Check sheet for the modelled part. Datum: model origin and axes. Units: mm. Face numbers are marked on the shaded views. A direction names the side the tool comes from. Round coordinates to 2 decimals unless told otherwise and drop trailing zeros. Write each loop counter-clockwise with the first axis right and the second up, starting at its lowest first coordinate (ties: lowest second). Pieces come first, ordered by that corner, then holes. Notation, with made-up numbers: (70.25, 2) -> (102.25, 2) arc R16 cw to (102.25, 20) -> close; hole circle Ø11 at (-34.75, 31). An arc over 180 degrees is marked (long way). Put each result on its own line as item: value. Start each with the question number.
from build123d import *

# Parameters (mm, degrees)
BOSS_EXTRUDE1_DEPTH                             = 6.35
SKETCH2_R                                       = 16.256
CUT_EXTRUDE1_DEPTH                              = 7.62
SKETCH3_R                                       = 10
CUT_EXTRUDE2_DEPTH                              = 31.770069873
CSK_FOR_M3_FLAT_HEAD_MACHINE_SCREW1_D           = 3.4
CSK_FOR_M3_FLAT_HEAD_MACHINE_SCREW1_CSINK_D     = 6.3
CSK_FOR_M3_FLAT_HEAD_MACHINE_SCREW1_CSINK_ANGLE = 90
CIRPATTERN1_COUNT                               = 4
F_8_32_TAPPED_HOLE1_D                           = 3.4544
F_8_32_TAPPED_HOLE1_DEPTH                       = 12.7
F_8_32_TAPPED_HOLE1_TIP                         = 1.037806461


with BuildPart() as part:
    # Sketch1 → Boss-Extrude1 (new, symmetric)
    with BuildSketch(Plane.XY):
        with BuildLine():
            Line((-21.08, 0), (-21.08, -17.78))
            Line((-21.08, -17.78), (21.08, -17.78))
            Line((21.08, -17.78), (21.08, 0))
            ThreePointArc((21.08, 0), (0, 21.08), (-21.08, 0))
        make_face()
    extrude(amount=BOSS_EXTRUDE1_DEPTH, both=True)

    # Sketch2 → Cut-Extrude1 (cut)
    with BuildSketch(Plane.XY.offset(6.35)):
        Circle(SKETCH2_R)
    extrude(amount=-CUT_EXTRUDE1_DEPTH, mode=Mode.SUBTRACT)

    # Sketch3 → Cut-Extrude2 (cut, through all)
    with BuildSketch(Plane.XY.offset(-1.27)):
        Circle(SKETCH3_R)
    extrude(amount=-CUT_EXTRUDE2_DEPTH, mode=Mode.SUBTRACT)

    # CSK for M3 Flat Head Machine Screw1 (through all)
    with Locations(Plane(origin=(0, 0, -6.35), x_dir=(-1, 0, 0), z_dir=(0, 0, -1))):
        with Locations((0, 13)):
            csk_for_m3_flat_head_machine_screw1 = CounterSinkHole(CSK_FOR_M3_FLAT_HEAD_MACHINE_SCREW1_D / 2, CSK_FOR_M3_FLAT_HEAD_MACHINE_SCREW1_CSINK_D / 2, counter_sink_angle=CSK_FOR_M3_FLAT_HEAD_MACHINE_SCREW1_CSINK_ANGLE)

    # CirPattern1: CSK for M3 Flat Head Machine Screw1 ×4 about axis
    cirpattern1_axis = Axis((0, 0, 0), (0, 0, 1))
    for i in range(1, CIRPATTERN1_COUNT):
        add(csk_for_m3_flat_head_machine_screw1.rotate(cirpattern1_axis, i * 360 / CIRPATTERN1_COUNT), mode=Mode.SUBTRACT)

    # #8-32 Tapped Hole1
    with Locations(Plane.XZ.offset(17.78)):
        with Locations((15.875, 0), (-15.875, 0)):
            Hole(F_8_32_TAPPED_HOLE1_D / 2, depth=F_8_32_TAPPED_HOLE1_DEPTH)
            with Locations((0, 0, -(F_8_32_TAPPED_HOLE1_DEPTH + F_8_32_TAPPED_HOLE1_TIP / 2))):  # 118° drill point
                Cone(0, F_8_32_TAPPED_HOLE1_D / 2, F_8_32_TAPPED_HOLE1_TIP, mode=Mode.SUBTRACT)


solid = part.part
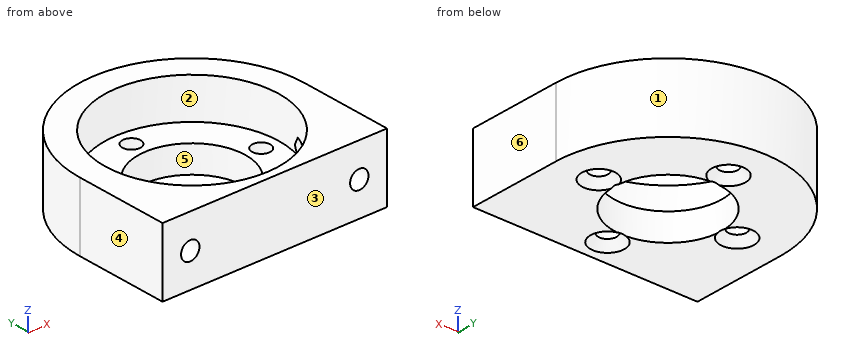
1. Material ranges on L1, parallel to Y at x = 0, z = -2.45; L2, parallel to X at y = -13, z = -3; L3, parallel to Y at x = 0, z = 4.5, recorded low to high. Write a range as [from, to].
2. Access from +Z, -Z, +X, -X, +Y, -Y to the whole of each face (thin tool, end or side, straight path). Record for the marked faces 1 and 2.
3. Draft check along X on the marked faces 3, 4, 5 and 6. Enter one of: released by +X, released by -X, zero draft, split by the parting line, or undercut.
4. Gauge pin test, flat ends, axial feed: P1, Ø4.5, axis at x = 15.875, z = 0, coming from the +Y side; P2, Ø2, axis at x = 0, y = 13, coming from the +Z side; P3, Ø1, axis at x = 5.5, y = -8.5, coming from the +Z side; P4, Ø12, axis at x = 8, y = 10.5, coming from the +Z side. Record the tip position at first contact, or that the pin passes through.
5. Section check D-D, the plane z = -3.5. Enter the section's corners in (x, y).
6. Section check C-C, the plane y = 9. Enter the section's corners in (x, z).
7. Section check A-A, the plane y = -13. Enter the section's corners in (x, z) (3 decimals).
8. Section check B-B, the plane x = 0. Enter the section's corners in (y, z).
Reply:
1. L1: y = [-17.78, -14.7], [-11.3, -10], [10, 11.3], [14.7, 21.08]
1. L2: x = [-21.08, -1.7], [1.7, 21.08]
1. L3: y = [-17.78, -16.26], [16.26, 21.08]
2. face 1: +Z, -Z, +Y
2. face 2: +Z
3. face 3: zero draft
3. face 4: released by -X
3. face 5: undercut
3. face 6: released by +X
4. P1: stops at y = 16.08
4. P2: passes through
4. P3: stops at z = -1.27
4. P4: stops at z = 6.35
5. outline: (-21.08, -17.78) -> (21.08, -17.78) -> (21.08, 0) arc R21.08 ccw to (-21.08, 0) -> close; hole circle Ø3.4 at (-13, 0); hole circle Ø20 at (0, 0); hole circle Ø3.4 at (0, -13); hole circle Ø3.4 at (0, 13); hole circle Ø3.4 at (13, 0)
6. outline: (-19.06, -6.35) -> (-4.36, -6.35) -> (-4.36, -1.27) -> (-13.54, -1.27) -> (-13.54, 6.35) -> (-19.06, 6.35) -> close; (4.36, -6.35) -> (19.06, -6.35) -> (19.06, 6.35) -> (13.54, 6.35) -> (13.54, -1.27) -> (4.36, -1.27) -> close
7. outline: (-21.08, -6.35) -> (-3.15, -6.35) -> (-1.7, -4.9) -> (-1.7, -1.27) -> (-9.76, -1.27) -> (-9.76, 6.35) -> (-21.08, 6.35) -> close; (1.7, -4.9) -> (3.15, -6.35) -> (21.08, -6.35) -> (21.08, 6.35) -> (9.76, 6.35) -> (9.76, -1.27) -> (1.7, -1.27) -> close; hole circle Ø3.454 at (-15.875, 0); hole circle Ø3.454 at (15.875, 0)
8. outline: (-17.78, -6.35) -> (-16.15, -6.35) -> (-14.7, -4.9) -> (-14.7, -1.27) -> (-16.26, -1.27) -> (-16.26, 6.35) -> (-17.78, 6.35) -> close; (-11.3, -4.9) -> (-10, -6.2) -> (-10, -1.27) -> (-11.3, -1.27) -> close; (10, -6.2) -> (11.3, -4.9) -> (11.3, -1.27) -> (10, -1.27) -> close; (14.7, -4.9) -> (16.15, -6.35) -> (21.08, -6.35) -> (21.08, 6.35) -> (16.26, 6.35) -> (16.26, -1.27) -> (14.7, -1.27) -> close
